Design review of the part built by this model. Coordinates are the model's own, in mm. Face numbers are marked on the shaded views. A direction names the side the tool comes from. Give positions to 0.01 mm unless a question says otherwise; leave off trailing zeros. Write each loop counter-clockwise with the first axis right and the second up, starting at its lowest first coordinate (ties: lowest second). Pieces come first, ordered by that corner, then holes. Notation, with made-up numbers: M -25.75,-31.75 L 9.25,-31.75 A27 cw 9.25,1.25 Z; hole C -6,-31 d10. An arc over 180 degrees is marked long. Answer in a Markdown table with one row per item.
```python
from build123d import *

# Parameters (mm, degrees)
F0_R          = 6.5
F1_DEPTH      = 5.1
F2_R          = 5
F3_DEPTH      = 6.15
F3_DEPTH_BACK = 1.05
F4_R          = 1.9
F5_DEPTH      = 7.3
F6_R          = 2.5
F7_DEPTH      = 2
F8_R          = 1.25
F9_DEPTH      = 13.4


with BuildPart() as f1:
    # F0 (on Top) → F1 (new body)
    with BuildSketch(Plane.XY):
        Circle(F0_R)
    extrude(amount=F1_DEPTH)

    # F2 (on Top) → F3 (join, two sides)
    with BuildSketch(Plane.XY) as f3_sk:
        Circle(F2_R)
    extrude(amount=F3_DEPTH)
    extrude(f3_sk.sketch, amount=-F3_DEPTH_BACK)

    # F4 (on Top) → F5 (join)
    with BuildSketch(Plane.XY):
        Circle(F4_R)
    extrude(amount=F5_DEPTH)

    # F6 (on Top) → F7 (join)
    with BuildSketch(Plane.XY):
        Circle(F6_R)
    extrude(amount=-F7_DEPTH)

    # F8 (on Top) → F9 (join)
    with BuildSketch(Plane.XY):
        Circle(F8_R)
    extrude(amount=F9_DEPTH)


solid = f1.part
```
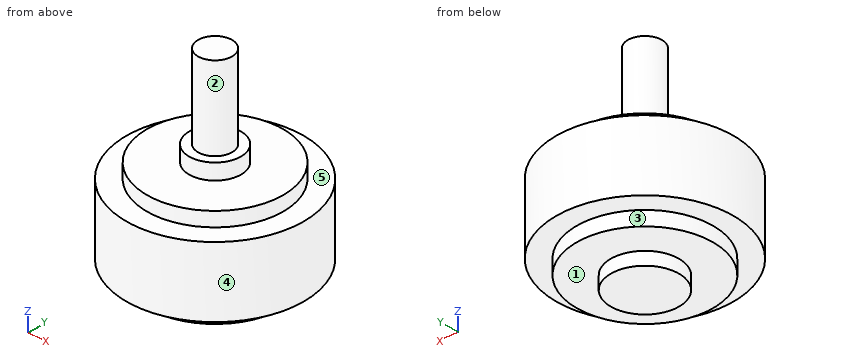
1) The part is to be moulded in two halves that separate along Y. For the marked faces 1 and 2, say which applies: released by +Y, released by -Y, zero draft, split by the parting line, or undercut.
Geometry says:
| item | result |
|---|---|
| face 1 | zero draft |
| face 2 | split by the parting line |
2) Add section A-A (x = 0). Write out the cut boundary in (y, z).
Geometry says:
| item | result |
|---|---|
| outline | M -6.5,0 L -5,0 L -5,-1.05 L -2.5,-1.05 L -2.5,-2 L 2.5,-2 L 2.5,-1.05 L 5,-1.05 L 5,0 L 6.5,0 L 6.5,5.1 L 5,5.1 L 5,6.15 L 1.9,6.15 L 1.9,7.3 L 1.25,7.3 L 1.25,13.4 L -1.25,13.4 L -1.25,7.3 L -1.9,7.3 L -1.9,6.15 L -5,6.15 L -5,5.1 L -6.5,5.1 Z |
3) For the marked faces 3, 4 and 5, list the 3-axis set-ups (+Z, -Z, +X, -X, +Y, -Y) from which the entire face can be reached by the end or side of a thin tool; tool diameter is ignored.
Geometry says:
| item | result |
|---|---|
| face 3 | -Z |
| face 4 | +Z, -Z |
| face 5 | +Z |
4) Add section C-C (z = 8.75). Write out the cut boundary in (x, y).
Geometry says:
| item | result |
|---|---|
| outline | C 0,0 d2.5 |
5) Add section B-B (y = -4.25). Write out the cut boundary in (x, z).
Geometry says:
| item | result |
|---|---|
| outline | M -4.92,0 L -2.63,0 L -2.63,-1.05 L 2.63,-1.05 L 2.63,0 L 4.92,0 L 4.92,5.1 L 2.63,5.1 L 2.63,6.15 L -2.63,6.15 L -2.63,5.1 L -4.92,5.1 Z |
6) Insertion check: P1, Ø3, axis at x = -2, y = 3.5, coming from the +Z side; P2, Ø3, axis at x = -2, y = -1.5, coming from the +Z side; P3, Ø1, axis at x = 2, y = 1, coming from the +Z side; P4, Ø1.5, axis at y = 2, z = 1.5, coming from the +X side. Each pin has a flat end and moves straight along its axis. Give the tip position at first contact, or say it passes through.
Geometry says:
| item | result |
|---|---|
| P1 | z = 6.15 |
| P2 | z = 13.4 |
| P3 | z = 7.3 |
| P4 | x = 6.38 |
7) To check wall thickness, follow probe 1 along Z at (x, y) = (3.25, 3.5); probe 2 along Z at (x, y) = (-1.5, 1); probe 3 along Y at (x, z) = (-2.75, 3.75). State the ranges of each line that lie inside material, in increasing order. Write a range as [from, to].
Geometry says:
| item | result |
|---|---|
| probe 1 | [-1.05, 6.15] |
| probe 2 | [-2, 7.3] |
| probe 3 | [-5.89, 5.89] |
